Study the drawing (mm; zero at the part's minimum x, y, z) and answer. Give positions to 0.01 mm unless a question says otherwise; leave off trailing zeros. Write each loop counter-clockwise with the first axis right and the second up, starting at its lowest first coordinate (ties: lowest second). Pieces come first, ordered by that corner, then holes. Notation, with made-up numbers: (50, -2.5) - (108, -2.5) arc R21 cw to (108, 7.5) - close; hole circle Ø6 at (9, 61). An arc over 180 degrees is marked (long way). Write each question's results on one line, items separated by ' | '. Start each with the question number.
Q1. Section A-A (z = 78.16) is taken. Determine the outline of the cut face in (x, y), plus the area to 3 significant figures.
Q2. Find the intervals of material crossed by probe 1 along X at (y, z) = (232.5, 78.16); probe 2 along X at (y, z) = (63, 78.16), in increasing order.
Q3. Section C-C (y = 80) is taken. Determine the outline of the cut face in (x, z).
Q4. For a pull along X with two mould halves and no side action, classify the marked faces 1, 2 and 3 as pulls with the +X half, pulls with the -X half, needs draft (parallel to the pull), parting line crosses it, or undercut.
Q5. Section D-D (y = 401) is taken. Determine the outline of the cut face in (x, z), plus the area to 3 significant figures.
Q6. Flat-ended cylindrical pins translate along their axes: pin 1 Ø1 at (y, z) = (279, 72) entering from +X; pin 2 Ø12 at (x, y) = (116, 86.5) entering from -Z; pin 3 Ø5 at (y, z) = (258.5, 105.5) entering from +X. Find the tip coordinate at first contact, or state that the pin passes through.
Q7. Section B-B (x = 78.16) is taken. Determine the outline of the cut face in (y, z).
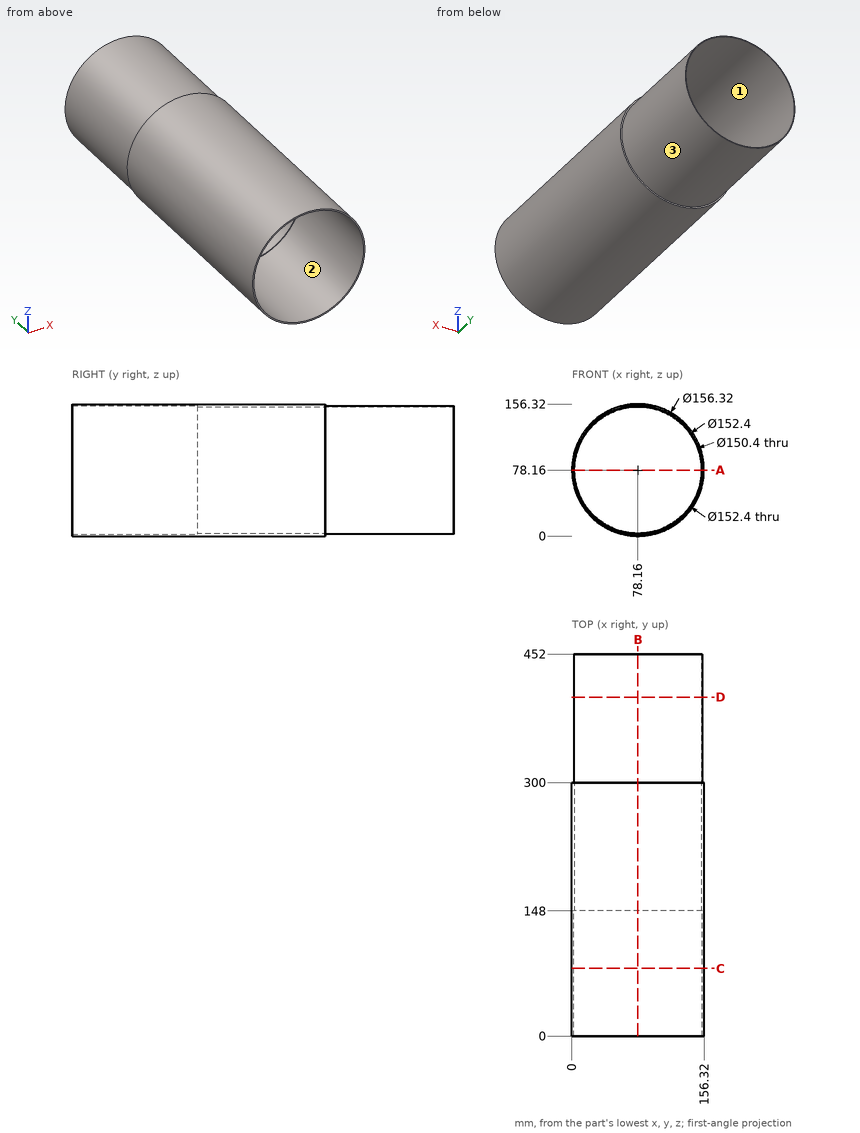
Answers below:
1) outline: (0, 0) - (1.96, 0) - (1.96, 148) - (2.96, 148) - (2.96, 452) - (1.96, 452) - (1.96, 300) - (0, 300) - close; (153.36, 148) - (154.36, 148) - (154.36, 0) - (156.32, 0) - (156.32, 300) - (154.36, 300) - (154.36, 452) - (153.36, 452) - close | area: 1,780 mm2
2) probe 1: x = 0 to 2.96, 153.36 to 156.32 | probe 2: x = 0 to 1.96, 154.36 to 156.32
3) outline: circle Ø156.32 at (78.16, 78.16); hole circle Ø152.4 at (78.16, 78.16)
4) face 1: undercut | face 2: undercut | face 3: parting line crosses it
5) outline: circle Ø152.4 at (78.16, 78.16); hole circle Ø150.4 at (78.16, 78.16) | area: 476 mm2
6) pin 1: stops at x = 156.11 | pin 2: stops at z = 6.78 | pin 3: stops at x = 152.27
7) outline: (0, 0) - (300, 0) - (300, 1.96) - (452, 1.96) - (452, 2.96) - (148, 2.96) - (148, 1.96) - (0, 1.96) - close; (0, 154.36) - (148, 154.36) - (148, 153.36) - (452, 153.36) - (452, 154.36) - (300, 154.36) - (300, 156.32) - (0, 156.32) - close
